CAD build for the part. Positions are in the model's coordinates, mm. Face numbers are marked on the shaded views. A direction names the side the tool comes from. Give positions to 0.01 mm unless a question says otherwise; leave off trailing zeros. Write each loop counter-clockwise with the first axis right and the second up, starting at its lowest first coordinate (ties: lowest second). Pieces come first, ordered by that corner, then holes. Notation, with made-up numbers: (76, 23.25) - (90, 23.25) arc R9 cw to (90, 34.25) - close; hole circle Ø6 at (-4, 31.5). An arc over 180 degrees is marked (long way). Answer as a JSON object with one key per item and string values.
from build123d import *

# Parameters (mm, degrees)
SKETCH1_R                 = 9.906
BOSS_EXTRUDE1_DEPTH       = 6.35
SKETCH2_W                 = 9.525
SKETCH2_H                 = 12.7
BOSS_EXTRUDE2_DEPTH       = 21.193
F_8_32_TAPPED_HOLE1_D     = 3.4544
F_8_32_TAPPED_HOLE1_DEPTH = 16.85544
F_8_32_TAPPED_HOLE1_TIP   = 1.037806461
FILLET1_R                 = 3.175


with BuildPart() as part:
    # Sketch1 → Boss-Extrude1 (new body)
    with BuildSketch(Plane.XY):
        with BuildLine():
            Line((7.675322169, 12.7), (0, 12.7))
            Line((0, 12.7), (0, 0))
            Line((0, 0), (7.675322169, 0))
            ThreePointArc((7.675322169, 0), (38.1, 6.35), (7.675322169, 12.7))
        make_face()
        with Locations((22.225, 6.35)):
            Circle(SKETCH1_R, mode=Mode.SUBTRACT)
    extrude(amount=BOSS_EXTRUDE1_DEPTH)

    # Sketch2 → Boss-Extrude2 (add)
    with BuildSketch(Plane.XY.offset(6.35)):
        with Locations((-4.7625, 6.35)):
            Rectangle(SKETCH2_W, SKETCH2_H)
    extrude(amount=-BOSS_EXTRUDE2_DEPTH)

    # #8-32 Tapped Hole1
    with Locations(Plane(origin=(0, 0, -14.843), x_dir=(-1, 0, 0), z_dir=(0, 0, -1))):
        with Locations((4.7625, 6.35)):
            Hole(F_8_32_TAPPED_HOLE1_D / 2, depth=F_8_32_TAPPED_HOLE1_DEPTH)
            with Locations((0, 0, -(F_8_32_TAPPED_HOLE1_DEPTH + F_8_32_TAPPED_HOLE1_TIP / 2))):  # 118° drill point
                Cone(0, F_8_32_TAPPED_HOLE1_D / 2, F_8_32_TAPPED_HOLE1_TIP, mode=Mode.SUBTRACT)

    # Fillet1
    fillet1_edges = [part.edges().sort_by_distance(p)[0] for p in [
        (0, 6.35, 0),
        (7.675322169, 12.7, 3.175),
        (7.675322169, 0, 3.175),
    ]]
    fillet(fillet1_edges, radius=FILLET1_R)


solid = part.part
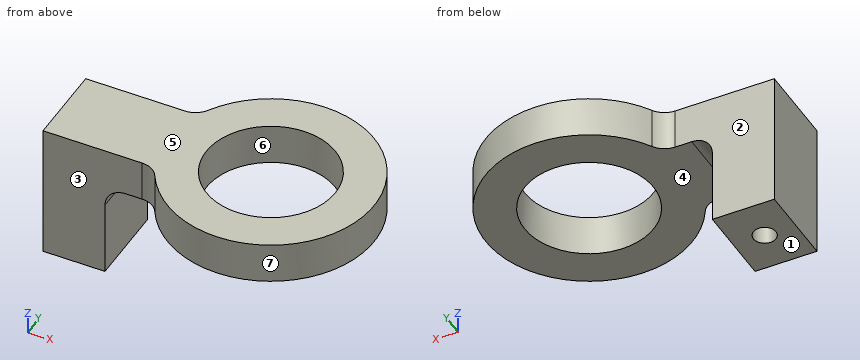
Item 1: Probe line 1 (X direction, y = 6.35, z = -7.5) (3 decimals); line 2 (Z direction, x = 31.5, y = 0); line 3 (X direction, y = 11, z = 2.25) (3 decimals). List the from-to ranges inside material, lowest first. Write a range as from..to.
Entries:
{"line 1": "-9.525..-6.49, -3.035..0", "line 2": "0..6.35", "line 3": "-9.525..13.478, 30.972..37.404"}
Item 2: Mould opens along Y. For the marked faces 5, 6 and 7 say: +Y half, -Y half, draft (parallel to the pull), parting line (faces both ways), or undercut.
Entries:
{"face 5": "draft", "face 6": "undercut", "face 7": "parting line"}
Item 3: Cut at D-D (y = 9). Give the cut face in (x, z) (3 decimals), and give its area (3 significant figures).
Entries:
{"outline": "(-9.525, -14.843) - (0, -14.843) - (0, -3.175) arc R3.175 cw to (3.175, 0) - (12.68, 0) - (12.68, 6.35) - (-9.525, 6.35) - close; (31.77, 0) - (37.877, 0) - (37.877, 6.35) - (31.77, 6.35) - close", "area": "323 mm2"}
Item 4: Flat gauge pins, fed straight in: P1, Ø1, axis at y = 12.5, z = -9, coming from the +X side; P2, Ø12, axis at x = 0.5, z = -3.5, coming from the -Y side; P3, Ø4.5, axis at x = -5, z = -4.5, coming from the +Y side; P4, Ø3, axis at x = 27, y = 0.5, coming from the +Z side (1 decimal). Where does each tip first touch, or does it go through?
Entries:
{"P1": "x = 0", "P2": "y = 0", "P3": "y = 12.7", "P4": "through"}
Item 5: Cut at B-B (y = 2). Give the cut face in (x, z) (3 decimals), and give its area (3 significant figures).
Entries:
{"outline": "(-9.525, -14.843) - (0, -14.843) - (0, -3.175) arc R3.175 cw to (3.175, 0) - (13.325, 0) - (13.325, 6.35) - (-9.525, 6.35) - close; (31.125, 0) - (37.492, 0) - (37.492, 6.35) - (31.125, 6.35) - close", "area": "329 mm2"}
Item 6: Cut at C-C (x = 17). Give the cut face in (y, z).
Entries:
{"outline": "(-8.64, 0) - (-2.07, 0) - (-2.07, 6.35) - (-8.64, 6.35) - close; (14.77, 0) - (21.34, 0) - (21.34, 6.35) - (14.77, 6.35) - close"}
Item 7: Which spindle directions (+Z, -Z, +X, -X, +Y, -Y) get a long thin tool onto all of the face, cutting with end or side? Do the marked faces 1, 2, 3 and 4. Say none if no direction does.
Entries:
{"face 1": "-Z, +X, -X, +Y, -Y", "face 2": "+Z, -Z, -X, +Y", "face 3": "+Z, -Z, -X, -Y", "face 4": "-Z, +X, +Y, -Y"}
